```python
from build123d import *

# Parameters (mm, degrees)
SKETCH1_W           = 64.5
SKETCH1_H           = 45.5
BOSS_EXTRUDE1_DEPTH = 2
SKETCH2_W           = 64.5
SKETCH2_H           = 45.5
SKETCH2_W_2         = 28
SKETCH2_H_2         = 41.5
BOSS_EXTRUDE2_DEPTH = 14
CUT_EXTRUDE1_REACH  = 80.565
SKETCH3_R           = 14
SKETCH4_W           = 2.5
SKETCH4_H           = 39.5
CUT_EXTRUDE2_DEPTH  = 5.5
SKETCH5_W           = 28
SKETCH5_H           = 41.5
BOSS_EXTRUDE3_DEPTH = 10.16
SKETCH6_R           = 1.2
BOSS_EXTRUDE4_DEPTH = 5.08


with BuildPart() as part:
    # Sketch1 → Boss-Extrude1 (new body)
    with BuildSketch(Plane(origin=(0, 0, 0), x_dir=(0, 0, -1), z_dir=(1, 0, 0))):
        with Locations((30.25, 20.75)):
            Rectangle(SKETCH1_W, SKETCH1_H)
    extrude(amount=BOSS_EXTRUDE1_DEPTH)

    # Sketch2 → Boss-Extrude2 (add)
    with BuildSketch(Plane.ZY):
        with Locations((-30.25, 20.75)):
            Rectangle(SKETCH2_W, SKETCH2_H)
        with Locations((-46.5, 20.75)):
            Rectangle(SKETCH2_W_2, SKETCH2_H_2, mode=Mode.SUBTRACT)
        with Locations((-14, 20.75)):
            Rectangle(SKETCH2_W_2, SKETCH2_H_2, mode=Mode.SUBTRACT)
    extrude(amount=BOSS_EXTRUDE2_DEPTH)

    # Sketch3 → Cut-Extrude1 (cut, up to next)
    with BuildSketch(Plane(origin=(0, -2, 0), x_dir=(1, 0, 0), z_dir=(0, 1, 0)), mode=Mode.PRIVATE) as cut_extrude1_sk1:
        with Locations((-14, 14)):
            Circle(SKETCH3_R)
    cut_extrude1_tool1 = extrude(cut_extrude1_sk1.sketch, amount=CUT_EXTRUDE1_REACH, mode=Mode.PRIVATE) & part.part
    add(cut_extrude1_tool1.solids().sort_by_distance((-14, -2, -14))[0], mode=Mode.SUBTRACT)

    # Sketch4 → Cut-Extrude2 (cut)
    with BuildSketch(Plane.ZY.offset(14)):
        with Locations((-30.25, 20.75)):
            Rectangle(SKETCH4_W, SKETCH4_H)
    extrude(amount=-CUT_EXTRUDE2_DEPTH, mode=Mode.SUBTRACT)

    # Sketch5 → Boss-Extrude3 (add)
    with BuildSketch(Plane.ZY):
        with Locations((-46.5, 20.75)):
            Rectangle(SKETCH5_W, SKETCH5_H)
    extrude(amount=BOSS_EXTRUDE3_DEPTH)

    # Sketch6 → Boss-Extrude4 (add)
    with BuildSketch(Plane(origin=(0, 0, -62.5), x_dir=(-1, 0, 0), z_dir=(0, 0, -1))):
        with Locations(Location((11.968, 10.7, 0), (0, 0, 180))):
            Circle(SKETCH6_R)
        with Locations(Location((11.968, 19.68025612, 0), (0, 0, 180))):
            Circle(SKETCH6_R)
    extrude(amount=BOSS_EXTRUDE4_DEPTH)


solid = part.part
```
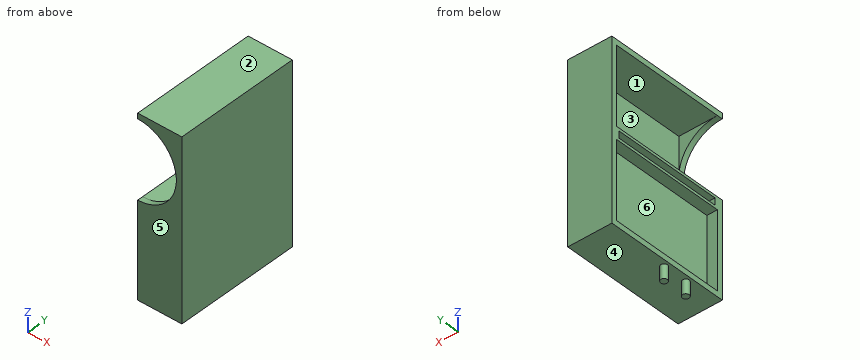
The listing builds one solid part. Answer for the finished solid, in the listing's coordinates (mm). Face numbers are marked on the shaded views. A direction names the side the tool comes from. Give positions to 0.01 mm unless a question says otherwise; leave off trailing zeros. Loops run counter-clockwise (first coordinate to the right, second up) from the corner with the lowest first, then second, coordinate; pieces in that order, holes last. Notation, with made-up numbers: M -6.75,-37 L 21.25,-37 A23 ccw 21.25,-2 Z; hole C 50,46 d3. An arc over 180 degrees is marked long. One line per item, written item: value.
Q1. A cutting plane is placed at D-D on z = -26. Determine the outline of the cut face in (x, y).
Working result:
outline: M -14,41.5 L 0,41.5 L 0,0 L -6.79,0 L -6.79,-2 L 2,-2 L 2,43.5 L -14,43.5 Z
Q2. A cutting plane is placed at B-B on z = -41. Determine the outline of the cut face in (x, y), then the cut area to 3 significant figures.
Working result:
outline: M -14,-2 L 2,-2 L 2,43.5 L -14,43.5 L -14,41.5 L -10.16,41.5 L -10.16,0 L -14,0 Z
area: 569 mm^2
Q3. A flat-ended cylindrical pin translates along its axis: P1, Ø8, axis at x = 0, y = 37.5, coming from the -Z side. Find the tip coordinate at first contact, or state that the pin passes through.
Working result:
P1: stops at z = -62.5
Q4. Determine the mould class of the marked faces 1, 2, 3 and 4 for opening direction Z: +Z half, -Z half, draft (parallel to the pull), parting line (faces both ways), or undercut.
Working result:
face 1: undercut
face 2: +Z half
face 3: undercut
face 4: -Z half
Q5. For the marked faces 5 and 6, determine the directions among +Z, -Z, +X, -X, +Y, -Y from which every point of the face is accessible in a straight line to the end or side of a thin tool.
Working result:
face 5: +Z, -Z, +X, -X, -Y
face 6: -X
Q6. Find the intervals of material crossed by line 1 (Z direction, x = -11.5, y = 11.5); line 2 (Z direction, x = -9.5, y = 9); line 3 (Z direction, x = -3, y = 18), in increasing order. Write a range as from..to.
Working result:
line 1: z = -67.58..-60.5, -32.5..-31.5, -29..-28, 0..2
line 2: z = -62.5..-31.5, -29..-28, 0..2
line 3: z = -62.5..-28, 0..2
Q7. A cutting plane is placed at C-C on x = -4.75. Determine the outline of the cut face in (y, z), then the cut area to 3 significant figures.
Working result:
outline: M -2,-62.5 L 43.5,-62.5 L 43.5,2 L -2,2 L -2,-3.49 L 0,-3.49 L 0,0 L 41.5,0 L 41.5,-28 L 0,-28 L 0,-24.51 L -2,-24.51 Z
area: 1,730 mm^2
Q8. A cutting plane is placed at A-A on y = 13.5. Determine the outline of the cut face in (x, z).
Working result:
outline: M -14,-62.5 L 2,-62.5 L 2,2 L -14,2 L -14,0 L 0,0 L 0,-28 L -14,-28 L -14,-29 L -8.5,-29 L -8.5,-31.5 L -14,-31.5 L -14,-32.5 L -10.16,-32.5 L -10.16,-60.5 L -14,-60.5 Z
